Drawing for the job (mm, zero at the part's lowest x, y, z). Give positions to 0.01 mm unless a question says otherwise; leave off trailing zeros. Loops run counter-clockwise (first coordinate to the right, second up) from the corner with the lowest first, then second, coordinate; pieces in that order, holes last. Notation, with made-up numbers: (65, -26) - (70, -26) arc R15 cw to (70, -7) - close; hole circle Ø5 at (-4.75, 82). An arc over 180 degrees is marked (long way). Return JSON: item names as keys, results as strings. Group by question number.
1) Slice it at B-B (x = 392.5). List the corners of the cut face in (y, z).
2) Drop flat-ended pins along their axis: pin 1 (4 mm diameter, centred on y = 7.5, z = 461, fed in from +X); pin 2 (6 mm diameter, centred on y = 14, z = 357, fed in from -X); pin 3 (2 mm diameter, centred on y = 11, z = 701.5, fed in from +X) (1 decimal). Give the stop position or say it passes through.
3) Drill centre lines: probe 1 along X at (y, z) = (7.25, 392.5); probe 2 along X at (y, z) = (5.75, 267.5); probe 3 along Z at (x, y) = (599.5, 6.5) (1 decimal). Where is each one in solid material? Low to high. Write a range as from..to.
4) Slice it at C-C (z = 239). List the corners of the cut face in (x, y), and give its area (3 significant figures).
5) Slice it at A-A (y = 4.5). List the corners of the cut face in (x, z), and give its area (3 significant figures).
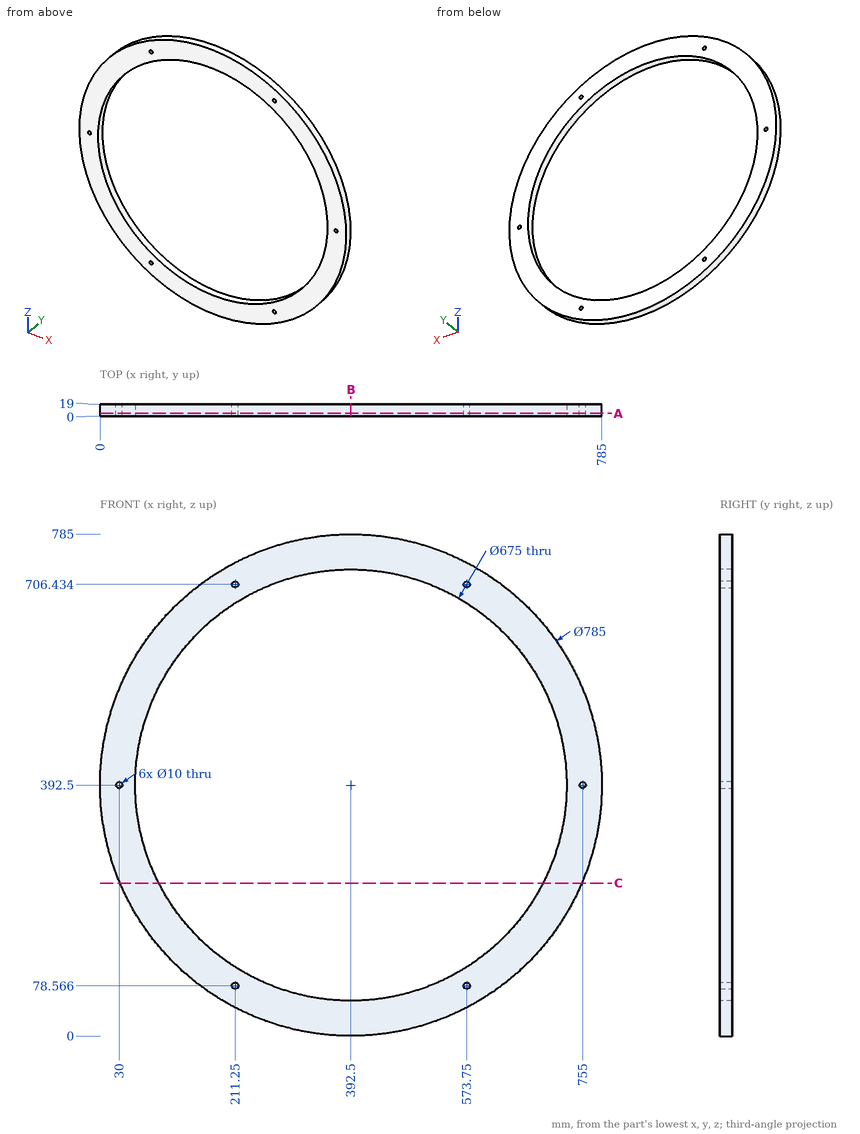
Results:
{
 "1": {"outline": "(0, 0) - (19, 0) - (19, 55) - (0, 55) - close; (0, 730) - (19, 730) - (19, 785) - (0, 785) - close"},
 "2": {"pin 1": "x = 779.33", "pin 2": "x = 1.35", "pin 3": "x = 635.8"},
 "3": {"probe 1": "0..25, 35..55, 730..750, 760..785", "probe 2": "20.44..79, 706..764.56", "probe 3": "59..125.9, 659.1..726"},
 "4": {"outline": "(31.26, 0) - (91.93, 0) - (91.93, 19) - (31.26, 19) - close; (693.07, 0) - (753.74, 0) - (753.74, 19) - (693.07, 19) - close", "area": "2,310 mm2"},
 "5": {"outline": "circle Ø785 at (392.5, 392.5); hole circle Ø10 at (30, 392.5); hole circle Ø675 at (392.5, 392.5); hole circle Ø10 at (211.25, 78.57); hole circle Ø10 at (211.25, 706.43); hole circle Ø10 at (573.75, 78.57); hole circle Ø10 at (573.75, 706.43); hole circle Ø10 at (755, 392.5)", "area": "126,000 mm2"}
}
